CAD build for the part. Positions are in the model's coordinates, mm. A direction names the side the tool comes from. Round coordinates to 2 decimals unless told otherwise and drop trailing zeros. Loops run counter-clockwise (first coordinate to the right, second up) from the corner with the lowest first, then second, coordinate; pieces in that order, holes last. Notation, with made-up numbers: (-18, 23.5) -> (6, 23.5) arc R30 ccw to (6, 55.5) -> close; hole circle Ø2 at (2.25, 29). An arc over 180 degrees is marked (long way). Answer as CSV lines item,"result".
```python
from build123d import *

# Parameters (mm, degrees)
SKETCH1_W           = 180.34
SKETCH1_H           = 167.64
CASE_2_DEPTH        = 38.1
SKETCH2_W           = 50.8
SKETCH2_H           = 25.4
TOP_HOLE_DEPTH      = 19.05
SKETCH3_W           = 19.05
SKETCH3_H           = 12.7
BOSS_EXTRUDE2_DEPTH = 2.54
SKETCH4_W           = 2.54
SKETCH4_H           = 8.89
BOSS_EXTRUDE3_DEPTH = 13.97
SKETCH5_R           = 1.905
CUT_EXTRUDE2_DEPTH  = 2.54
SKETCH6_W           = 19.05
SKETCH6_H           = 12.7
BOSS_EXTRUDE4_DEPTH = 2.54


with BuildPart() as part:
    # Sketch1 → case 2 (new body, symmetric)
    with BuildSketch(Plane.XY):
        with Locations((90.17, 83.82)):
            Rectangle(SKETCH1_W, SKETCH1_H)
    extrude(amount=CASE_2_DEPTH, both=True)

    # Sketch2 → top hole (cut)
    with BuildSketch(Plane(origin=(0, 167.64, 0), x_dir=(1, 0, 0), z_dir=(0, 1, 0))):
        with Locations((25.4, -25.4)):
            Rectangle(SKETCH2_W, SKETCH2_H)
        with Locations((154.94, -25.4)):
            Rectangle(SKETCH2_W, SKETCH2_H)
    extrude(amount=-TOP_HOLE_DEPTH, mode=Mode.SUBTRACT)

    # Sketch3 → Boss-Extrude2 (add)
    with BuildSketch(Plane(origin=(0, 148.59, 0), x_dir=(1, 0, 0), z_dir=(0, 1, 0))):
        with Locations((15.875, -25.4)):
            Rectangle(SKETCH3_W, SKETCH3_H)
    extrude(amount=BOSS_EXTRUDE2_DEPTH)

    # Sketch4 → Boss-Extrude3 (add)
    with BuildSketch(Plane(origin=(0, 151.13, 0), x_dir=(1, 0, 0), z_dir=(0, 1, 0))):
        with Locations((20.32, -25.4)):
            Rectangle(SKETCH4_W, SKETCH4_H)
    boss_extrude3 = extrude(amount=BOSS_EXTRUDE3_DEPTH)

    # Sketch5 → Cut-Extrude2 (cut)
    with BuildSketch(Plane(origin=(21.59, 0, 0), x_dir=(0, 0, -1), z_dir=(1, 0, 0))):
        with BuildLine():
            ThreePointArc((-22.225, 165.1), (-21.326974388, 164.728025612), (-20.955, 163.83))
            Line((-20.955, 163.83), (-20.955, 165.1))
            Line((-20.955, 165.1), (-22.225, 165.1))
        make_face()
        with BuildLine():
            Line((-29.845, 165.1), (-29.845, 163.83))
            ThreePointArc((-29.845, 163.83), (-29.473025612, 164.728025612), (-28.575, 165.1))
            Line((-28.575, 165.1), (-29.845, 165.1))
        make_face()
        with Locations((-25.4, 160.02)):
            Circle(SKETCH5_R)
    cut_extrude2 = extrude(amount=-CUT_EXTRUDE2_DEPTH, mode=Mode.SUBTRACT)

    # Sketch6 → Boss-Extrude4 (add)
    with BuildSketch(Plane(origin=(0, 148.59, 0), x_dir=(1, 0, 0), z_dir=(0, 1, 0))):
        with Locations((164.465, -25.4)):
            Rectangle(SKETCH6_W, SKETCH6_H)
    extrude(amount=BOSS_EXTRUDE4_DEPTH)

    # Mirror1: Boss-Extrude3, Cut-Extrude2 across plane
    add(boss_extrude3.mirror(Plane(origin=(90.17, 0, 0), x_dir=(0, 0, 1), z_dir=(1, 0, 0))))
    add(cut_extrude2.mirror(Plane(origin=(90.17, 0, 0), x_dir=(0, 0, 1), z_dir=(1, 0, 0))), mode=Mode.SUBTRACT)


solid = part.part
```
Q1. Slice it at B-B, the plane x = 139. Give the cut face in (y, z).
Results:
outline,"(0, -38.1) -> (167.64, -38.1) -> (167.64, 12.7) -> (148.59, 12.7) -> (148.59, 38.1) -> (0, 38.1) -> close"
Q2. Probe L1, parallel to Z at x = 159.9, y = 160.02 (3 decimals); L2, parallel to X at y = 154.5, z = 28.5; L3, parallel to Y at x = 20, z = 25. List the from-to ranges inside material, lowest first. Write a range as [from, to].
Results:
L1,"[-38.1, 12.7], [20.955, 23.495], [27.305, 29.845]"
L2,"[19.05, 21.59], [50.8, 129.54], [158.75, 161.29]"
L3,"[0, 158.16], [161.88, 165.1]"
Q3. Slice it at A-A, the plane x = 11. Give the cut face in (y, z).
Results:
outline,"(0, -38.1) -> (167.64, -38.1) -> (167.64, 12.7) -> (148.59, 12.7) -> (148.59, 19.05) -> (151.13, 19.05) -> (151.13, 31.75) -> (148.59, 31.75) -> (148.59, 38.1) -> (0, 38.1) -> close"
Q4. Drop flat-ended pins along their axis: pin 1 Ø2 at (y, z) = (150.5, 23.5) entering from -X; pin 2 Ø7.5 at (x, z) = (162, 31) entering from +Y; pin 3 Ø21 at (y, z) = (162.5, 31.5) entering from +X. Give the stop position or say it passes through.
Results:
pin 1,"x = 6.35"
pin 2,"y = 165.1"
pin 3,"x = 161.29"
Q5. Tool access for faces 1 (the flat face through (25, 158, 12.7)), 2 (the flat face through (158.75, 158, 25)), 3 (the flat face through (161.29, 158, 25)), 4 (the flat face through (19.05, 158, 25)): list every direction of +Z, -Z, +X, -X, +Y, -Y with a clear straight run to the whole face (end or side of a thin tool).
Results:
face 1,"-X, +Y"
face 2,"+Z, +Y"
face 3,"+Z, +X, +Y"
face 4,"+Z, -X, +Y"
Q6. Two-plate mould, pull along Z, no slides. Class faces 5 (the flat face through (89, 85, 38.1)), 6 (the flat face through (21.59, 158, 25)), 7 (the flat face through (89, 85, -38.1)), 8 (the flat face through (31, 148.59, 25)): pulls with the +Z half, pulls with the -Z half, needs draft (parallel to the pull), parting line crosses it, or undercut.
Results:
face 5,"pulls with the +Z half"
face 6,"needs draft"
face 7,"pulls with the -Z half"
face 8,"undercut"
